For this review, take the finished solid that the model builds, in its own axes (mm). Give positions to 0.01 mm unless a question says otherwise; leave off trailing zeros. Order: outer loops, then holes, each group sorted by start corner. A loop starts at its lowest first (then second) coordinate and runs counter-clockwise, first axis right, second up.
Item 1: Consider section A-A (x = -457). Give the boundary of the cut face in (y, z), plus the area to 3 significant figures.
Item 2: For probe 1 along Z at (x, y) = (312.5, 17); probe 2 along X at (y, z) = (82.5, 208.5); probe 3 along Z at (x, y) = (-829, 76.5), list the stretches that pass through material, from the lowest coordinate up.
Item 3: For P1, Ø1.5, axis at x = -959, z = 216, coming from the +Y side; P2, Ø2.5, axis at x = -252.5, y = 1, coming from the +Z side; P3, Ø18.5, axis at x = -945, z = 419.5, coming from the +Y side, all flat-tipped, find the tip position at first contact; note any pin that passes through.
```python
from build123d import *

# Parameters (mm, degrees)
SKETCH1_W           = 1920
SKETCH1_H           = 1994
BOSS_EXTRUDE1_DEPTH = 120
SKETCH2_W           = 60
SKETCH2_H           = 60
CUT_EXTRUDE1_DEPTH  = 2167.750793239
SKETCH3_W           = 40
SKETCH3_H           = 40
CUT_EXTRUDE2_DEPTH  = 2167.750793239
SKETCH4_W           = 1920
SKETCH4_H           = 40
CUT_EXTRUDE3_DEPTH  = 3
SKETCH5_W           = 40
SKETCH5_H           = 1874
CUT_EXTRUDE4_DEPTH  = 3
SKETCH6_W           = 1874
SKETCH6_H           = 40
CUT_EXTRUDE5_DEPTH  = 3


with BuildPart() as part:
    # Sketch1 → Boss-Extrude1 (new body)
    with BuildSketch(Plane(origin=(0, 0, 0), x_dir=(1, 0, 0), z_dir=(0, 1, 0))):
        Rectangle(SKETCH1_W, SKETCH1_H)
    extrude(amount=BOSS_EXTRUDE1_DEPTH)

    # Sketch2 → Cut-Extrude1 (cut, through all)
    with BuildSketch(Plane.ZY.offset(960)):
        with Locations((-967, 90)):
            Rectangle(SKETCH2_W, SKETCH2_H)
        with Locations((967, 90)):
            Rectangle(SKETCH2_W, SKETCH2_H)
    extrude(amount=-CUT_EXTRUDE1_DEPTH, mode=Mode.SUBTRACT)

    # Sketch3 → Cut-Extrude2 (cut, through all)
    with BuildSketch(Plane.ZY.offset(960)):
        with Locations((0, 20)):
            Rectangle(SKETCH3_W, SKETCH3_H)
    extrude(amount=-CUT_EXTRUDE2_DEPTH, mode=Mode.SUBTRACT)

    # Sketch4 → Cut-Extrude3 (cut)
    with BuildSketch(Plane(origin=(0, 0, 0), x_dir=(-1, 0, 0), z_dir=(0, -1, 0))):
        with Locations((0, 977)):
            Rectangle(SKETCH4_W, SKETCH4_H)
        with Locations((0, -977)):
            Rectangle(SKETCH4_W, SKETCH4_H)
    extrude(amount=-CUT_EXTRUDE3_DEPTH, mode=Mode.SUBTRACT)

    # Sketch5 → Cut-Extrude4 (cut)
    with BuildSketch(Plane(origin=(0, 120, 0), x_dir=(1, 0, 0), z_dir=(0, 1, 0))):
        with Locations((-940, 0)):
            Rectangle(SKETCH5_W, SKETCH5_H)
        with Locations((940, 0)):
            Rectangle(SKETCH5_W, SKETCH5_H)
    extrude(amount=-CUT_EXTRUDE4_DEPTH, mode=Mode.SUBTRACT)

    # Sketch6 → Cut-Extrude5 (cut)
    with BuildSketch(Plane.ZY.offset(960)):
        with Locations((0, 100)):
            Rectangle(SKETCH6_W, SKETCH6_H)
    cut_extrude5 = extrude(amount=-CUT_EXTRUDE5_DEPTH, mode=Mode.SUBTRACT)

    # Mirror1: Cut-Extrude5 across plane
    add(cut_extrude5.mirror(Plane(origin=(0, 0, 0), x_dir=(0, 0, 1), z_dir=(1, 0, 0))), mode=Mode.SUBTRACT)


solid = part.part
```
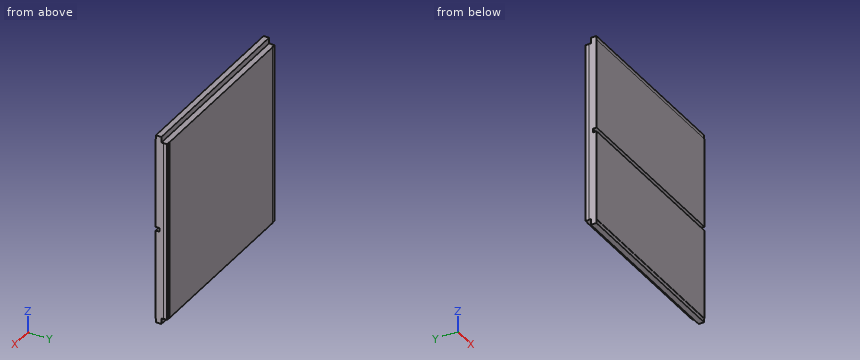
Resolved:
1. outline: (0, -957) - (3, -957) - (3, -997) - (60, -997) - (60, -937) - (120, -937) - (120, 937) - (60, 937) - (60, 997) - (3, 997) - (3, 957) - (0, 957) - (0, 20) - (40, 20) - (40, -20) - (0, -20) - close
1. area: 230,000 mm2
2. probe 1: z = -997 to -20, 20 to 997
2. probe 2: x = -957 to 957
2. probe 3: z = -937 to 937
3. P1: stops at y = 80
3. P2: stops at z = 957
3. P3: stops at y = 117
